```python
from build123d import *

# Parameters (mm, degrees)
SKETCH2_W            = 114.3
SKETCH2_H            = 63.5
BOSS_EXTRUDE1_DEPTH  = 6.35
SKETCH3_R            = 1.75
CUT_EXTRUDE1_DEPTH   = 7.35
SKETCH4_W            = 63.5
SKETCH4_H            = 63.5
BOSS_EXTRUDE2_DEPTH  = 6.35
SKETCH5_R            = 1.75
CUT_EXTRUDE2_DEPTH   = 7.35
LPATTERN1_COUNT      = 8
LPATTERN1_PITCH      = 8
LPATTERN1_COUNT_DIR2 = 4
LPATTERN1_PITCH_DIR2 = 8
LPATTERN2_COUNT      = 8
LPATTERN2_PITCH      = 8
LPATTERN2_COUNT_DIR2 = 4
LPATTERN2_PITCH_DIR2 = 8
SKETCH6_W            = 38.1
SKETCH6_H            = 38.1
CUT_EXTRUDE3_DEPTH   = 7.35
FILLET1_R            = 2.54


with BuildPart() as part:
    # Sketch2 → Boss-Extrude1 (new body)
    with BuildSketch(Plane.XY):
        with Locations((57.15, 31.75)):
            Rectangle(SKETCH2_W, SKETCH2_H)
    extrude(amount=BOSS_EXTRUDE1_DEPTH)

    # Sketch3 → Cut-Extrude1 (cut, through all)
    with BuildSketch(Plane.XY.offset(6.35)):
        with Locations((25.4, 31.75)):
            Circle(SKETCH3_R)
        with Locations((105.4, 31.75)):
            Circle(SKETCH3_R)
        with Locations((6.35, 57.15)):
            Circle(SKETCH3_R)
        with Locations((6.35, 6.35)):
            Circle(SKETCH3_R)
        with Locations((107.95, 6.35)):
            Circle(SKETCH3_R)
        with Locations((107.95, 57.15)):
            Circle(SKETCH3_R)
    extrude(amount=-CUT_EXTRUDE1_DEPTH, mode=Mode.SUBTRACT)

    # Sketch4 → Boss-Extrude2 (add, through all)
    with BuildSketch(Plane.XY.offset(6.35)):
        with Locations((146.05, 31.75)):
            Rectangle(SKETCH4_W, SKETCH4_H)
    extrude(amount=-BOSS_EXTRUDE2_DEPTH)

    # Sketch5 → Cut-Extrude2 (cut, through all)
    with BuildSketch(Plane.XY.offset(6.35)):
        with Locations((113.4, 31.75)):
            Circle(SKETCH5_R)
    cut_extrude2 = extrude(amount=-CUT_EXTRUDE2_DEPTH, mode=Mode.SUBTRACT)

    # LPattern1: Cut-Extrude2 8 × 4
    with Locations(*[(i * LPATTERN1_PITCH, -j * LPATTERN1_PITCH_DIR2, 0) for i in range(LPATTERN1_COUNT) for j in range(LPATTERN1_COUNT_DIR2) if (i, j) != (0, 0)]):
        add(cut_extrude2, mode=Mode.SUBTRACT)

    # LPattern2: Cut-Extrude2 8 × 4
    with Locations(*[(i * LPATTERN2_PITCH, j * LPATTERN2_PITCH_DIR2, 0) for i in range(LPATTERN2_COUNT) for j in range(LPATTERN2_COUNT_DIR2) if (i, j) != (0, 0)]):
        add(cut_extrude2, mode=Mode.SUBTRACT)

    # Sketch6 → Cut-Extrude3 (cut, through all)
    with BuildSketch(Plane.XY.offset(6.35)):
        with Locations((65.4, 31.75)):
            Rectangle(SKETCH6_W, SKETCH6_H)
    extrude(amount=-CUT_EXTRUDE3_DEPTH, mode=Mode.SUBTRACT)

    # Fillet1
    fillet1_edges = [part.edges().sort_by_distance(p)[0] for p in [
        (46.35, 12.7, 3.175),
        (46.35, 50.8, 3.175),
        (84.45, 50.8, 3.175),
        (84.45, 12.7, 3.175),
    ]]
    fillet(fillet1_edges, radius=FILLET1_R)


solid = part.part
```
Here's how the part is built. I have some questions about the finished solid (model axes, mm). Coordinates: 2 decimals unless noted, no trailing zeros. Write each loop counter-clockwise with the first axis right and the second up, starting at its lowest first coordinate (ties: lowest second). Pieces come first, ordered by that corner, then holes. Notation, with made-up numbers: M 68.5,54 L 79.5,54 A13 cw 79.5,67 Z; hole C 19,-2.5 d9. An arc over 180 degrees is marked long. Answer as CSV lines item,"result". Start each with the question number.
Q1. I need wall thicknesses on probe 1 along Y at (x, z) = (73.5, 5.25); probe 2 along X at (y, z) = (35, 2); probe 3 along Y at (x, z) = (25, 5.75). Which ranges of each line are inside material? Lowest first, please. Write a range as [from, to].
Q2. Suppose I cut it at B-B, the plane x = 66. List the corners of the cut face in (y, z) for me, then the cut area to 3 significant figures.
Q3. Suppose I cut it at A-A, the plane x = 129.4. State how many separate pieces and enclosed holes the cut face has, then the cut area to 3 significant figures.
Entries:
1,probe 1,"y = [0, 12.7], [50.8, 63.5]"
1,probe 2,"x = [0, 46.35], [84.45, 177.8]"
1,probe 3,"y = [0, 30.05], [33.45, 63.5]"
2,outline,"M 0,0 L 12.7,0 L 12.7,6.35 L 0,6.35 Z; M 50.8,0 L 63.5,0 L 63.5,6.35 L 50.8,6.35 Z"
2,area,"161 mm²"
3,separate pieces,"8"
3,enclosed holes,"0"
3,area,"248 mm²"
